```python
from build123d import *
from build123d.topology import SkipClean

# Parameters (mm, degrees)
SKETCH1_R               = 3.25
BOSS_EXTRUDE1_DEPTH     = 13.7
SKETCH2_W               = 42.3
SKETCH2_H               = 42.3
SKETCH2_R               = 11.25
BOSS_EXTRUDE2_DEPTH     = 2
CUT_EXTRUDE1_DEPTH      = 33.898860163
SKETCH4_R               = 1.75
CUT_EXTRUDE2_DEPTH      = 33.898860163
MIRROR6_COPY_1_SKETCH_R = 1.75
MIRROR6_COPY_1_DEPTH    = 33.898860163
BOSS_EXTRUDE3_DEPTH     = 2
CUT_EXTRUDE3_DEPTH      = 2
FILLET1_R               = 2


with BuildPart() as part:
    # Sketch1 → Boss-Extrude1 (new body)
    with BuildSketch(Plane(origin=(0, 0, 0), x_dir=(1, 0, 0), z_dir=(0, 1, 0))):
        with Locations(Location((-15.5, 15.5, 0), (0, 0, 270))):
            Circle(SKETCH1_R)
    extrude(amount=BOSS_EXTRUDE1_DEPTH)


with BuildPart() as body_2:
    # Mirror2: mirrored copy
    add(part.part.mirror(Plane(origin=(0, 0, 0), x_dir=(0, 0, 1), z_dir=(1, 0, 0))))


with BuildPart() as body_3:
    # Mirror3: mirrored copy
    add(part.part.mirror(Plane.XY))


with BuildPart() as body_4:
    # Mirror3 2: mirrored copy
    add(body_2.part.mirror(Plane.XY))


with BuildPart() as part_1:
    add(part.part)

    add(body_2.part)  # Boss-Extrude2 merges body 2

    add(body_3.part)  # Boss-Extrude2 merges body 3

    add(body_4.part)  # Boss-Extrude2 merges body 4
    # Sketch2 → Boss-Extrude2 (add)
    with BuildSketch(Plane(origin=(0, 13.7, 0), x_dir=(1, 0, 0), z_dir=(0, 1, 0))):
        Rectangle(SKETCH2_W, SKETCH2_H)
        with Locations(Location((0, 0, 0), (0, 0, 270))):
            Circle(SKETCH2_R, mode=Mode.SUBTRACT)
    extrude(amount=-BOSS_EXTRUDE2_DEPTH)

    # Sketch3 → Cut-Extrude1 (cut, through all)
    with BuildSketch(Plane(origin=(0, 13.7, 0), x_dir=(1, 0, 0), z_dir=(0, 1, 0))):
        Polygon((-16.963055506, 21.15), (-21.15, 16.963055506), (-21.15, 21.15), align=None)
        Polygon((16.963055506, -21.15), (21.15, -16.963055506), (21.15, -21.15), align=None)
    cut_extrude1 = extrude(amount=-CUT_EXTRUDE1_DEPTH, mode=Mode.SUBTRACT)

    # Mirror4: Cut-Extrude1 across plane
    add(cut_extrude1.mirror(Plane.XY), mode=Mode.SUBTRACT)

    # Sketch4 → Cut-Extrude2 (cut, through all)
    with BuildSketch(Plane.XZ):
        with Locations(Location((15.5, -15.5, 0), (0, 0, 270))):
            Circle(SKETCH4_R)
    cut_extrude2 = extrude(amount=-CUT_EXTRUDE2_DEPTH, mode=Mode.SUBTRACT)

    # Mirror5: Cut-Extrude2 across plane
    add(cut_extrude2.mirror(Plane(origin=(0, 0, 0), x_dir=(0, 0, 1), z_dir=(1, 0, 0))), mode=Mode.SUBTRACT)

    # Mirror6: Cut-Extrude2 across plane
    add(cut_extrude2.mirror(Plane.XY), mode=Mode.SUBTRACT)

    # Mirror6 copy 1 sketch → Mirror6 copy 1 (cut, through all)
    with BuildSketch(Plane(origin=(0, 0, 0), x_dir=(-1, 0, 0), z_dir=(0, -1, 0))):
        with Locations(Location((15.5, -15.5, 0), (0, 0, 270))):
            Circle(MIRROR6_COPY_1_SKETCH_R)
    extrude(amount=-MIRROR6_COPY_1_DEPTH, mode=Mode.SUBTRACT)

    # Sketch6 → Boss-Extrude3 (add)
    with SkipClean():  # the faces are left unmerged after this step: merging them gives an invalid solid
        with BuildSketch(Plane.XZ.offset(-11.7)):
            with BuildLine():
                Line((-3, -21.15), (-3, -10.842624221))
                ThreePointArc((-3, -10.842624221), (0, -11.25), (3, -10.842624221))
                Line((3, -10.842624221), (3, -21.15))
                Line((3, -21.15), (-3, -21.15))
            make_face()
        extrude(amount=BOSS_EXTRUDE3_DEPTH)

    # Sketch7 → Cut-Extrude3 (cut)
    with SkipClean():  # the faces are left unmerged after this step: merging them gives an invalid solid
        with BuildSketch(Plane(origin=(0, 13.7, 0), x_dir=(1, 0, 0), z_dir=(0, 1, 0))):
            with BuildLine():
                Line((-1, 11.25), (-1, 21.15))
                ThreePointArc((-1, 21.15), (0, 22.15), (1, 21.15))
                Line((1, 21.15), (1, 11.25))
                ThreePointArc((1, 11.25), (0, 10.25), (-1, 11.25))
            make_face()
        extrude(amount=-CUT_EXTRUDE3_DEPTH, mode=Mode.SUBTRACT)

    # Fillet1
    fillet1_edges = [part_1.edges().sort_by_distance(p)[0] for p in [
        (3, 9.7, -15.996312111),
        (-3, 9.7, -15.996312111),
    ]]
    fillet(fillet1_edges, radius=FILLET1_R - 0.0001)  # a hair under: the kernel refuses the full size


solid = part_1.part
```
Could you check a few things on this model? Use its own coordinates, in mm. A direction names the side the tool comes from. Round coordinates to 2 decimals unless told otherwise and drop trailing zeros. Loops run counter-clockwise (first coordinate to the right, second up) from the corner with the lowest first, then second, coordinate; pieces in that order, holes last. Notation, with made-up numbers: (3.25, 66.5) - (7.25, 66.5) arc R17 cw to (7.25, 74.5) - close; hole circle Ø2 at (73.5, 54). An arc over 180 degrees is marked (long way). Answer in a Markdown table with one row per item. Add a question column.
(1) I need wall thicknesses on line 1 along X through (y, z) = (3.5, -15.5); line 2 along X through (y, z) = (12.9, 0); line 3 along Z through (x, y) = (-16, 1.5). Which ranges of each line are inside material? Lowest first, please.
(2) If we section it at C-C (z = 15.5): Please give me the cut outline in (x, y), plus the area to 3 significant figures.
(3) For faces 5 (the face through (0, 11, -21.15)), 6 (the face through (-12.278, 5.768, -15.923)), 7 (the face through (-1, 13, -16)), which set-ups out of +Z, -Z, +X, -X, +Y, -Y let a thin tool reach every point of the face, with its end or its side?
(4) I'm going to push flat-ended pins straight in: pin 1 (1.6 mm diameter, centred on x = 0, z = -15.5, fed in from -Y); pin 2 (0.6 mm diameter, centred on x = 0.5, z = -14.5, fed in from +Y). Where does each tip first touch, or does it pass through?
(5) If we section it at B-B (x = -15.5): Please give me the cut outline in (y, z).
(6) If we section it at D-D (y = 7.5): Please give me the cut outline in (x, z).
(7) If we section it at A-A (y = 10.25): State how many separate pieces and enclosed holes the cut face has, plus the area to 3 significant figures.
(8) If we mould it in two halves opening along Z, with no side actions, what happens to faces 1 (the face through (12.278, 5.768, -15.923)), 2 (the face through (-19.027, 12.714, -19.086)), 3 (the face through (-19.027, 12.714, 19.086)), 4 (the face through (2.43, 10.3, -16.07))? For each: pulls with the +Z half, pulls with the -Z half, needs draft (parallel to the pull), parting line crosses it, or undercut.
Model answer:
| question | item | result |
|---|---|---|
| 1 | line 1 | x = -18.75 to -17.25, -13.75 to -12.25, 12.25 to 13.75, 17.25 to 18.75 |
| 1 | line 2 | x = -21.15 to -11.25, 11.25 to 21.15 |
| 1 | line 3 | z = -18.71 to -17.18, -13.82 to -12.29, 12.29 to 13.82, 17.18 to 18.71 |
| 2 | outline | (-21.15, 11.7) - (-18.75, 11.7) - (-18.75, 0) - (-17.25, 0) - (-17.25, 13.7) - (-21.15, 13.7) - close; (-13.75, 0) - (-12.25, 0) - (-12.25, 11.7) - (12.25, 11.7) - (12.25, 0) - (13.75, 0) - (13.75, 13.7) - (-13.75, 13.7) - close; (17.25, 0) - (18.75, 0) - (18.75, 11.7) - (21.15, 11.7) - (21.15, 13.7) - (17.25, 13.7) - close |
| 2 | area | 141 mm² |
| 3 | face 5 | -Z, +X, -X, +Y, -Y |
| 3 | face 6 | -Y |
| 3 | face 7 | -Z, +Y |
| 4 | pin 1 | stops at y = 9.7 |
| 4 | pin 2 | stops at y = 11.7 |
| 5 | outline | (0, -18.75) - (11.7, -18.75) - (11.7, -21.15) - (13.7, -21.15) - (13.7, -17.25) - (0, -17.25) - close; (0, -13.75) - (13.7, -13.75) - (13.7, 13.75) - (0, 13.75) - (0, 12.25) - (11.7, 12.25) - (11.7, -12.25) - (0, -12.25) - close; (0, 17.25) - (13.7, 17.25) - (13.7, 21.15) - (11.7, 21.15) - (11.7, 18.75) - (0, 18.75) - close |
| 6 | outline | circle Ø6.5 at (-15.5, -15.5); circle Ø6.5 at (-15.5, 15.5); circle Ø6.5 at (15.5, -15.5); circle Ø6.5 at (15.5, 15.5); hole circle Ø3.5 at (-15.5, -15.5); hole circle Ø3.5 at (-15.5, 15.5); hole circle Ø3.5 at (15.5, -15.5); hole circle Ø3.5 at (15.5, 15.5) |
| 7 | separate pieces | 5 |
| 7 | enclosed holes | 4 |
| 7 | area | 142 mm² |
| 8 | face 1 | undercut |
| 8 | face 2 | pulls with the -Z half |
| 8 | face 3 | pulls with the +Z half |
| 8 | face 4 | needs draft |
